Geometry check sheet. Reference: the model listing, model coordinates, mm. A direction names the side the tool comes from. Coordinates: 2 decimals unless noted, no trailing zeros. Loops run counter-clockwise (first coordinate to the right, second up) from the corner with the lowest first, then second, coordinate; pieces in that order, holes last. Notation, with made-up numbers: M 84.25,51.5 L 122.25,51.5 A5 cw 122.25,57.5 Z; hole C -19,15.5 d1. An arc over 180 degrees is marked long. Use CSV: the item, a comma, the result in double quotes.
```python
from build123d import *
from build123d.topology import SkipClean

# Parameters (mm, degrees)
SKETCH1_R               = 32
BOSS_EXTRUDE1_DEPTH     = 5
BOSS_EXTRUDE4_DEPTH     = 20
SKETCH5_R               = 32
BOSS_EXTRUDE5_DEPTH     = 5
CUT_EXTRUDE1_DEPTH      = 52.701063819
CUT_EXTRUDE1_DEPTH_BACK = 5
SKETCH2_7_R             = 2.9
SKETCH1_3_R             = 22
CUT_EXTRUDE2_DEPTH      = 10
SKETCH6_R               = 4.9
BOSS_EXTRUDE7_DEPTH     = 25
FILLET1_R               = 5


with BuildPart() as part:
    # Sketch1 → Boss-Extrude1 (new body)
    with BuildSketch(Plane(origin=(0, 0, 0), x_dir=(1, 0, 0), z_dir=(0, 1, 0))):
        with Locations(Location((0, 0, 0), (0, 0, 270))):
            Circle(SKETCH1_R)
    extrude(amount=BOSS_EXTRUDE1_DEPTH)

    # Sketch2 → Boss-Extrude4 (add)
    with SkipClean():  # the faces are left unmerged after this step: merging them gives an invalid solid
        with BuildSketch(Plane(origin=(0, 5, 0), x_dir=(1, 0, 0), z_dir=(0, 1, 0))):
            with BuildLine():
                Line((-23.592874778, 21.618886644), (-22.118320104, 20.267706228))
                ThreePointArc((-22.118320104, 20.267706228), (-21.213203436, 21.213203436), (-20.267706228, 22.118320104))
                Line((-20.267706228, 22.118320104), (-21.618886644, 23.592874778))
                ThreePointArc((-21.618886644, 23.592874778), (-22.627416998, 22.627416998), (-23.592874778, 21.618886644))
            make_face()
            with BuildLine():
                Line((23.592874778, 21.618886644), (22.118320104, 20.267706228))
                ThreePointArc((22.118320104, 20.267706228), (21.213203436, 21.213203436), (20.267706228, 22.118320104))
                Line((20.267706228, 22.118320104), (21.618886644, 23.592874778))
                ThreePointArc((21.618886644, 23.592874778), (22.627416998, 22.627416998), (23.592874778, 21.618886644))
            make_face()
            with BuildLine():
                Line((21.618886644, -23.592874778), (20.267706228, -22.118320104))
                ThreePointArc((20.267706228, -22.118320104), (21.213203436, -21.213203436), (22.118320104, -20.267706228))
                Line((22.118320104, -20.267706228), (23.592874778, -21.618886644))
                ThreePointArc((23.592874778, -21.618886644), (22.627416998, -22.627416998), (21.618886644, -23.592874778))
            make_face()
            with BuildLine():
                Line((-23.592874778, -21.618886644), (-22.118320104, -20.267706228))
                ThreePointArc((-22.118320104, -20.267706228), (-21.213203436, -21.213203436), (-20.267706228, -22.118320104))
                Line((-20.267706228, -22.118320104), (-21.618886644, -23.592874778))
                ThreePointArc((-21.618886644, -23.592874778), (-22.627416998, -22.627416998), (-23.592874778, -21.618886644))
            make_face()
        extrude(amount=BOSS_EXTRUDE4_DEPTH)

    # Sketch5 → Boss-Extrude5 (add)
    with SkipClean():  # the faces are left unmerged after this step: merging them gives an invalid solid
        with BuildSketch(Plane(origin=(0, 25, 0), x_dir=(1, 0, 0), z_dir=(0, 1, 0))):
            with Locations(Location((0, 0, 0), (0, 0, 270))):
                Circle(SKETCH5_R)
        extrude(amount=BOSS_EXTRUDE5_DEPTH)

    # Sketch2_7 → Cut-Extrude1 (cut, two sides: drawn at the far end of the back side and taken through both)
    with SkipClean():  # the faces are left unmerged after this step: merging them gives an invalid solid
        with BuildSketch(Plane(origin=(0, 5, 0), x_dir=(1, 0, 0), z_dir=(0, 1, 0)).offset(-CUT_EXTRUDE1_DEPTH_BACK)):
            with Locations(Location((27, 0, 0), (0, 0, 270))):
                Circle(SKETCH2_7_R)
            with Locations(Location((0, -27, 0), (0, 0, 270))):
                Circle(SKETCH2_7_R)
            with Locations(Location((0, 27, 0), (0, 0, 270))):
                Circle(SKETCH2_7_R)
            with Locations(Location((-27, 0, 0), (0, 0, 270))):
                Circle(SKETCH2_7_R)
        extrude(amount=CUT_EXTRUDE1_DEPTH + CUT_EXTRUDE1_DEPTH_BACK, mode=Mode.SUBTRACT)

    # Sketch1_3 → Cut-Extrude2 (cut)
    with SkipClean():  # the faces are left unmerged after this step: merging them gives an invalid solid
        with BuildSketch(Plane(origin=(0, 0, 0), x_dir=(1, 0, 0), z_dir=(0, 1, 0))):
            with Locations(Location((0, 0, 0), (0, 0, 270))):
                Circle(SKETCH1_3_R)
        extrude(amount=CUT_EXTRUDE2_DEPTH, mode=Mode.SUBTRACT)

    # Sketch6 → Boss-Extrude7 (add)
    with SkipClean():  # the faces are left unmerged after this step: merging them gives an invalid solid
        with BuildSketch(Plane(origin=(0, 30, 0), x_dir=(1, 0, 0), z_dir=(0, 1, 0))):
            with Locations(Location((0, 0, 0), (0, 0, 270))):
                Circle(SKETCH6_R)
        extrude(amount=BOSS_EXTRUDE7_DEPTH)

    # Fillet1
    fillet1_edges = [part.edges().sort_by_distance(p)[0] for p in [
        (0, 30, -4.9),
    ]]
    fillet(fillet1_edges, radius=FILLET1_R)


solid = part.part
```
1. Section check A-A, the plane x = 0. Count the separate pieces of the cut face and the enclosed holes in it, plus the area to 3 significant figures.
The answers:
separate pieces,"7"
enclosed holes,"0"
area,"560 mm^2"
2. Release check for a two-part mould opening along Z. For faces 5 (the cylindrical face through (24.17, 27.46, -0.63)), 6 (the flat face through (8, 0, 21)), 7 (the cylindrical face through (1.472, 44.86, 4.674)) record: +Z half, -Z half, draft (parallel to the pull), parting line (faces both ways), or undercut.
The answers:
face 5,"undercut"
face 6,"draft"
face 7,"parting line"
3. Gauge pin test, flat ends, axial feed: P1, Ø3, axis at x = -9.5, y = 28, coming from the -Z side; P2, Ø7.5, axis at x = -27, z = 0, coming from the +Y side; P3, Ø12, axis at x = 22.5, y = 40.5, coming from the -Z side; P4, Ø3, axis at y = 24.5, z = -23, coming from the +X side. Record the tip position at first contact, or that the pin passes through.
The answers:
P1,"z = -30.98"
P2,"y = 30"
P3,"through"
P4,"x = 23.62"
4. Set-up check for faces 1 (the cylindrical face through (-1.11, 27.46, -24.32)), 2 (the flat face through (-19, 5, -12)), 3 (the flat face through (-7, 30, -8)), 4 (the cylindrical face through (-21.477, 2.465, -4.769)): record each of +Z, -Z, +X, -X, +Y, -Y from which the full face is reachable in a straight line by a thin tool's end or side.
The answers:
face 1,"+Y, -Y"
face 2,"none"
face 3,"+Y"
face 4,"-Y"
5. Thickness scan on line 1 (Z direction, x = 0, y = 1.4); line 2 (Z direction, x = 0, y = 26.4). Record the ranges inside material, lowest first. Write a range as [from, to].
The answers:
line 1,"[-32, -29.9], [-24.1, -22], [22, 24.1], [29.9, 32]"
line 2,"[-32, -29.9], [-24.1, 24.1], [29.9, 32]"
6. Section check B-B, the plane y = 10. Record the cut outline in (x, z).
The answers:
outline,"M -23.59,-21.62 A32 ccw -21.62,-23.59 L -20.27,-22.12 A30 cw -22.12,-20.27 Z; M -23.59,21.62 L -22.12,20.27 A30 cw -20.27,22.12 L -21.62,23.59 A32 ccw Z; M 20.27,-22.12 L 21.62,-23.59 A32 ccw 23.59,-21.62 L 22.12,-20.27 A30 cw Z; M 20.27,22.12 A30 cw 22.12,20.27 L 23.59,21.62 A32 ccw 21.62,23.59 Z"
7. Section check C-C, the plane z = -12. Record the cut outline in (x, y).
The answers:
outline,"M -29.66,0 L -18.44,0 L -18.44,5 L -29.66,5 Z; M -29.66,25 L 29.66,25 L 29.66,30 L -29.66,30 Z; M 18.44,0 L 29.66,0 L 29.66,5 L 18.44,5 Z"
8. Section check D-D, the plane x = -15. Record the cut outline in (y, z), plus the area to 3 significant figures.
The answers:
outline,"M 0,-28.27 L 5,-28.27 L 5,-16.09 L 0,-16.09 Z; M 0,16.09 L 5,16.09 L 5,28.27 L 0,28.27 Z; M 25,-28.27 L 30,-28.27 L 30,28.27 L 25,28.27 Z"
area,"404 mm^2"
